```python
from build123d import *

# Parameters (mm, degrees)
BOSS_EXTRUDE3_DEPTH = 30


with BuildPart() as part:
    # Sketch1 → Boss-Extrude3 (new body)
    with BuildSketch(Plane.XY):
        with BuildLine():
            ThreePointArc((-10, 47.018073759), (-14.854364506, 45.717033096), (-19.546360403, 43.916273236))
            add(Edge.make_bspline(
                [(-19.546360403, 43.916273236), (-113.09637125, 140.200566945), (-121.402656368, 218.135469823)],
                knots=[0, 0, 0, 1, 1, 1], degree=2, weights=[1, 2.333333333, 1]))
            ThreePointArc((-121.402656368, 218.135469823), (-130.070701563, 213.080503011), (-138.528602909, 207.681280679))
            add(Edge.make_bspline(
                [(-35.72670029, 32.160568191), (-127.721013505, 141.647594866), (-138.528602909, 207.681280679)],
                knots=[0, 0, 0, 1, 1, 1], degree=2, weights=[1, 3, 1]))
            ThreePointArc((-35.72670029, 32.160568191), (-38.889231158, 28.254680318), (-41.626675488, 24.039948997))
            add(Edge.make_bspline(
                [(-41.626675488, 24.039948997), (-173.904711956, 46.948262171), (-226.433624328, 105.116611161)],
                knots=[0, 0, 0, 1, 1, 1], degree=2, weights=[1, 2.333333333, 1]))
            ThreePointArc((-226.433624328, 105.116611161), (-230.474985255, 95.932107972), (-234.14398792, 86.592615672))
            add(Edge.make_bspline(
                [(-47.807015375, 5.018818671), (-186.586837749, 39.522783313), (-234.14398792, 86.592615672)],
                knots=[0, 0, 0, 1, 1, 1], degree=2, weights=[1, 3, 1]))
            ThreePointArc((-47.807015375, 5.018818671), (-48.069733304, 0), (-47.807015375, -5.018818671))
            add(Edge.make_bspline(
                [(-47.807015375, -5.018818671), (-168.2873635, -64.236683039), (-244.974643991, -48.053220183)],
                knots=[0, 0, 0, 1, 1, 1], degree=2, weights=[1, 2.333333333, 1]))
            ThreePointArc((-244.974643991, -48.053220183), (-242.845658137, -57.8590917), (-240.324327808, -67.571485346))
            add(Edge.make_bspline(
                [(-41.626675488, -24.039948997), (-174.182831827, -77.698388136), (-240.324327808, -67.571485346)],
                knots=[0, 0, 0, 1, 1, 1], degree=2, weights=[1, 3, 1]))
            ThreePointArc((-41.626675488, -24.039948997), (-38.889231158, -28.254680318), (-35.72670029, -32.160568191))
            add(Edge.make_bspline(
                [(-35.72670029, -32.160568191), (-98.389962063, -150.885398653), (-169.943676031, -182.868354686)],
                knots=[0, 0, 0, 1, 1, 1], degree=2, weights=[1, 2.333333333, 1]))
            ThreePointArc((-169.943676031, -182.868354686), (-162.457543631, -189.5500849), (-154.708942796, -195.925575633))
            add(Edge.make_bspline(
                [(-19.546360403, -43.916273236), (-95.246904403, -165.241416188), (-154.708942796, -195.925575633)],
                knots=[0, 0, 0, 1, 1, 1], degree=2, weights=[1, 3, 1]))
            ThreePointArc((-19.546360403, -43.916273236), (-14.854364506, -45.717033096), (-10, -47.018073759))
            add(Edge.make_bspline(
                [(-10, -47.018073759), (9.08906073, -179.901020388), (-30, -247.833993165)],
                knots=[0, 0, 0, 1, 1, 1], degree=2, weights=[1, 2.333333333, 1]))
            ThreePointArc((-30, -247.833993165), (-20.016169186, -248.839388239), (-10, -249.442755293))
            add(Edge.make_bspline(
                [(10, -47.018073759), (20.070103179, -189.667839605), (-10, -249.442755293)],
                knots=[0, 0, 0, 1, 1, 1], degree=2, weights=[1, 3, 1]))
            ThreePointArc((10, -47.018073759), (14.854364506, -45.717033096), (19.546360403, -43.916273236))
            add(Edge.make_bspline(
                [(19.546360403, -43.916273236), (113.09637125, -140.200566945), (121.402656368, -218.135469823)],
                knots=[0, 0, 0, 1, 1, 1], degree=2, weights=[1, 2.333333333, 1]))
            ThreePointArc((121.402656368, -218.135469823), (130.070701563, -213.080503011), (138.528602909, -207.681280679))
            add(Edge.make_bspline(
                [(35.72670029, -32.160568191), (127.721013505, -141.647594866), (138.528602909, -207.681280679)],
                knots=[0, 0, 0, 1, 1, 1], degree=2, weights=[1, 3, 1]))
            ThreePointArc((35.72670029, -32.160568191), (38.889231158, -28.254680318), (41.626675488, -24.039948997))
            add(Edge.make_bspline(
                [(41.626675488, -24.039948997), (173.904711956, -46.948262171), (226.433624328, -105.116611161)],
                knots=[0, 0, 0, 1, 1, 1], degree=2, weights=[1, 2.333333333, 1]))
            ThreePointArc((226.433624328, -105.116611161), (230.474985255, -95.932107972), (234.14398792, -86.592615672))
            add(Edge.make_bspline(
                [(47.807015375, -5.018818671), (186.586837749, -39.522783313), (234.14398792, -86.592615672)],
                knots=[0, 0, 0, 1, 1, 1], degree=2, weights=[1, 3, 1]))
            ThreePointArc((47.807015375, -5.018818671), (48.069733304, 0), (47.807015375, 5.018818671))
            add(Edge.make_bspline(
                [(47.807015375, 5.018818671), (168.2873635, 64.236683039), (244.974643991, 48.053220183)],
                knots=[0, 0, 0, 1, 1, 1], degree=2, weights=[1, 2.333333333, 1]))
            ThreePointArc((244.974643991, 48.053220183), (242.845658137, 57.8590917), (240.324327808, 67.571485346))
            add(Edge.make_bspline(
                [(41.626675488, 24.039948997), (174.182831827, 77.698388136), (240.324327808, 67.571485346)],
                knots=[0, 0, 0, 1, 1, 1], degree=2, weights=[1, 3, 1]))
            ThreePointArc((41.626675488, 24.039948997), (38.889231158, 28.254680318), (35.72670029, 32.160568191))
            add(Edge.make_bspline(
                [(35.72670029, 32.160568191), (98.389962063, 150.885398653), (169.943676031, 182.868354686)],
                knots=[0, 0, 0, 1, 1, 1], degree=2, weights=[1, 2.333333333, 1]))
            ThreePointArc((169.943676031, 182.868354686), (162.457543631, 189.5500849), (154.708942796, 195.925575633))
            add(Edge.make_bspline(
                [(19.546360403, 43.916273236), (95.246904403, 165.241416188), (154.708942796, 195.925575633)],
                knots=[0, 0, 0, 1, 1, 1], degree=2, weights=[1, 3, 1]))
            ThreePointArc((19.546360403, 43.916273236), (14.854364506, 45.717033096), (10, 47.018073759))
            add(Edge.make_bspline(
                [(10, 47.018073759), (-9.08906073, 179.901020388), (30, 247.833993165)],
                knots=[0, 0, 0, 1, 1, 1], degree=2, weights=[1, 2.333333333, 1]))
            ThreePointArc((30, 247.833993165), (20.016169186, 248.839388239), (10, 249.442755293))
            add(Edge.make_bspline(
                [(-10, 47.018073759), (-20.070103179, 189.667839605), (10, 249.442755293)],
                knots=[0, 0, 0, 1, 1, 1], degree=2, weights=[1, 3, 1]))
        make_face()
    extrude(amount=BOSS_EXTRUDE3_DEPTH)


solid = part.part
```
CAD build for the part. Positions are in the model's coordinates, mm. Round coordinates to 2 decimals unless told otherwise and drop trailing zeros. Answer in a Markdown table with one row per item. Add a question column.
Item 1: Drill centre lines: line 1 (Y direction, x = -82, z = 23.5); line 2 (Y direction, x = -104, z = 27.5); line 3 (X direction, y = 82.5, z = 1). Where is each one in solid material? Low to high. Write a range as from..to.
Item 2: Drop flat-ended pins along their axis: pin 1 Ø1 at (y, z) = (-144, 15) entering from -X; pin 2 Ø3 at (y, z) = (-177.5, 23.5) entering from +X; pin 3 Ø8 at (x, z) = (9.5, 6) entering from -Y. Give the stop position or say it passes through.
Item 3: Saw through at A-A, the plane x = 84. Count the separate pieces of the cut face and the enclosed holes in it, then the cut area to 3 significant figures.
Findings below:
| question | item | result |
|---|---|---|
| 1 | line 1 | y = -139.95..-114.17, -40.25..-21.56, 13.6..31.32, 87.94..111.74 |
| 1 | line 2 | y = -164.65..-142.45, -48.89..-31.76, 19.25..35.69, 116.06..144.21 |
| 1 | line 3 | x = -229.99..-204.84, -77.58..-56.3, -12.43..5.11, 43.78..63.01 |
| 2 | pin 1 | stops at x = -106.06 |
| 2 | pin 2 | stops at x = 133.23 |
| 2 | pin 3 | stops at y = -216.22 |
| 3 | separate pieces | 4 |
| 3 | enclosed holes | 0 |
| 3 | area | 2,560 mm^2 |
